from build123d import *

# Parameters (mm, degrees)
F0_R     = 30.48
F1_DEPTH = 25.4
F2_R     = 26.67
F3_DEPTH = 60.96
F4_R     = 9.525
F5_DEPTH = 50.8


with BuildPart() as f1:
    # F0 (on Front) → F1 (new body)
    with BuildSketch(Plane.XZ):
        Circle(F0_R)
    extrude(amount=F1_DEPTH)

    # F2 (on face) → F3 (join)
    with BuildSketch(Plane.XZ.offset(25.4)):
        Circle(F2_R)
    extrude(amount=F3_DEPTH)

    # F4 (on Right) → F5 (join)
    with BuildSketch(Plane.YZ):
        with Locations((-48.26, -17.042583)):
            Circle(F4_R)
    extrude(amount=F5_DEPTH)


solid = f1.part
Can you work these out from the model? Positions are in its coordinate system, mm. A direction names the side the tool comes from. Coordinates: 2 decimals unless noted, no trailing zeros. Loops run counter-clockwise (first coordinate to the right, second up) from the corner with the lowest first, then second, coordinate; pieces in that order, holes last. Notation, with made-up numbers: (-27.5, 25.5) - (25.5, 25.5) arc R9 ccw to (25.5, 34.5) - close; hole circle Ø5 at (46, 63.5). An arc over 180 degrees is marked (long way). Put each result on its own line as item: value. Start each with the question number.
Item 1: Suppose I cut it at C-C (y = -59). Please give me the cut outline in (x, z), and give its area (3 significant figures).
Item 2: For pin 1 (8 mm diameter, centred on x = 7, y = -69.5, fed in from +Z); pin 2 (6 mm diameter, centred on x = -6.5, y = -10, fed in from -Z); pin 3 (6 mm diameter, centred on x = -5, y = -26.5, fed in from +Z), each with a flat end and sliding along its axis, tell me the tip position at first contact or that it passes through.
Item 3: Suppose I cut it at A-A (z = 0). Please give me the cut outline in (x, y), and give its area (3 significant figures).
Item 4: Suppose I cut it at D-D (x = 25). Please give me the cut outline in (y, z) (3 decimals), and give its area (3 significant figures).
Item 5: Which directions (+Z, -Z, +X, -X, +Y, -Y) give clear straight access to the entire face, cutting with the end or side of a thin tool? Please do faces 5 (the face through (31.606, -50.325, -26.341)), 6 (the face through (50.8, -48, -17)).
Item 6: Suppose I cut it at B-B (x = 0). Please give me the cut outline in (y, z).
Item 7: If we mould it in two halves opening along Y, with no side actions, what happens to faces 1 (the face through (0, -86.36, 0)), 2 (the face through (0, -25.4, -27)), 3 (the face through (-6.607, -12.522, -29.755)), 4 (the face through (0, 0, 0))? For each: +Y half, -Y half, draft (parallel to the pull), parting line (faces both ways), or undercut.
Item 8: If I drill on line 1 along Y through (x, z) = (-15.5, 22); line 2 along X through (y, z) = (-72, -24.5); line 3 along X through (y, z) = (-61, -1), over which ranges is the centre line in solid material (lowest first)?
Here are the results:
1. outline: circle Ø53.34 at (0, 0)
1. area: 2,230 mm²
2. pin 1: z = 26.5
2. pin 2: z = -30.28
2. pin 3: z = 30.4
3. outline: (-30.48, -25.4) - (-26.67, -25.4) - (-26.67, -86.36) - (26.67, -86.36) - (26.67, -25.4) - (30.48, -25.4) - (30.48, 0) - (-30.48, 0) - close
3. area: 4,800 mm²
4. outline: (-86.36, -9.289) - (-53.793, -9.289) arc R9.525 ccw (long way) to (-42.727, -9.289) - (-25.4, -9.289) - (-25.4, -17.436) - (0, -17.436) - (0, 17.436) - (-25.4, 17.436) - (-25.4, 9.289) - (-86.36, 9.289) - close
4. area: 2,290 mm²
5. face 5: +X
5. face 6: +Z, -Z, +X, +Y, -Y
6. outline: (-86.36, -26.67) - (-25.4, -26.67) - (-25.4, -30.48) - (0, -30.48) - (0, 30.48) - (-25.4, 30.48) - (-25.4, 26.67) - (-86.36, 26.67) - close
7. face 1: -Y half
7. face 2: undercut
7. face 3: draft
7. face 4: +Y half
8. line 1: -25.4 to 0
8. line 2: -10.54 to 10.54
8. line 3: -26.65 to 26.65
